```python
from build123d import *

# Parameters (mm, degrees)
BOSS_EXTRUDE1_DEPTH = 48
SKETCH2_R           = 1.5
CUT_EXTRUDE1_DEPTH  = 13
SKETCH3_R           = 1.5
SKETCH3_R_2         = 3
CUT_EXTRUDE3_DEPTH  = 21
FILLET1_R           = 5
FILLET2_R           = 15


with BuildPart() as part:
    # Sketch1 → Boss-Extrude1 (new body)
    with BuildSketch(Plane(origin=(0, 0, 0), x_dir=(1, 0, 0), z_dir=(0, 1, 0))):
        Polygon((0, 0), (0, 12), (1.5, 12), (1.5, 1.5), (20, 1.5), (20, 0), align=None)
    extrude(amount=BOSS_EXTRUDE1_DEPTH)

    # Sketch2 → Cut-Extrude1 (cut, through all)
    with BuildSketch(Plane.XY):
        with Locations((13, 31.5)):
            Circle(SKETCH2_R)
        with Locations((13, 16.5)):
            Circle(SKETCH2_R)
    extrude(amount=-CUT_EXTRUDE1_DEPTH, mode=Mode.SUBTRACT)

    # Sketch3 → Cut-Extrude3 (cut, through all)
    with BuildSketch(Plane(origin=(0, 0, 0), x_dir=(0, 0, -1), z_dir=(1, 0, 0))):
        with Locations((7, 42)):
            Circle(SKETCH3_R)
        with Locations((7, 24)):
            Circle(SKETCH3_R_2)
        with Locations((7, 6)):
            Circle(SKETCH3_R)
    extrude(amount=CUT_EXTRUDE3_DEPTH, mode=Mode.SUBTRACT)

    # Fillet1
    fillet1_edges = [part.edges().sort_by_distance(p)[0] for p in [
        (0.75, 48, -12),
        (0.75, 0, -12),
    ]]
    fillet(fillet1_edges, radius=FILLET1_R)

    # Fillet2
    fillet2_edges = [part.edges().sort_by_distance(p)[0] for p in [
        (20, 48, -0.75),
        (20, 0, -0.75),
    ]]
    fillet(fillet2_edges, radius=FILLET2_R)


solid = part.part
```
Verification items for the finished model (mm, model axes). A direction names the side the tool comes from. Coordinates: 2 decimals unless noted, no trailing zeros. Write each loop counter-clockwise with the first axis right and the second up, starting at its lowest first coordinate (ties: lowest second). Pieces come first, ordered by that corner, then holes. Notation, with made-up numbers: M 6,-4.75 L 45,-4.75 A28 cw 45,22.25 Z; hole C 75.25,-7 d1. An arc over 180 degrees is marked long. One line per item, written item: value.
Item 1: Section check A-A, the plane y = 31.5. Record the boundary of the cut face in (x, z), plus the area to 4 significant figures.
Check sheet entries:
outline: M 0,-12 L 1.5,-12 L 1.5,-1.5 L 11.5,-1.5 L 11.5,0 L 0,0 Z; M 14.5,-1.5 L 20,-1.5 L 20,0 L 14.5,0 Z
area: 41.25 mm^2
Item 2: Mould release check, pull along Z, two halves, no side actions. Record for faces 1 (the flat face through (11, 24, -1.5)), 2 (the cylindrical face through (0.74, 40.536, -6.675)), 3 (the cylindrical face through (15.49, 43.72, -0.74)): pulls with the +Z half, pulls with the -Z half, needs draft (parallel to the pull), parting line crosses it, or undercut.
Check sheet entries:
face 1: pulls with the -Z half
face 2: undercut
face 3: needs draft
Item 3: Gauge pin test, flat ends, axial feed: pin 1 Ø12 at (x, y) = (11, 26) entering from -Z; pin 2 Ø1.5 at (x, z) = (3.5, -9) entering from +Y; pin 3 Ø5 at (y, z) = (35, -6) entering from +X. Record the tip position at first contact, or that the pin passes through.
Check sheet entries:
pin 1: stops at z = -1.5
pin 2: passes through
pin 3: stops at x = 1.5
Item 4: Section check B-B, the plane x = 13. Record the boundary of the cut face in (y, z), plus the area to 3 significant figures.
Check sheet entries:
outline: M 2.31,-1.5 L 15,-1.5 L 15,0 L 2.31,0 Z; M 18,-1.5 L 30,-1.5 L 30,0 L 18,0 Z; M 33,-1.5 L 45.69,-1.5 L 45.69,0 L 33,0 Z
area: 56.1 mm^2
Item 5: Access from +Z, -Z, +X, -X, +Y, -Y to the whole of each face (thin tool, end or side, straight path). Record for faces 4 (the cylindrical face through (1, 1, -10)), 5 (the flat face through (1.5, 24, -3)).
Check sheet entries:
face 4: -Z, +X, -X, -Y
face 5: -Z, +X, +Y, -Y
Item 6: Scan lines: line 1 along Y through (x, z) = (0.7, -7); line 2 along Y through (x, z) = (1, -8.25); line 3 along Y through (x, z) = (13, -0.55). Record each from-to range of solid material in increasing order.
Check sheet entries:
line 1: y = 0 to 4.5, 7.5 to 21, 27 to 40.5, 43.5 to 48
line 2: y = 0.16 to 5.17, 6.83 to 21.27, 26.73 to 41.17, 42.83 to 47.84
line 3: y = 2.31 to 15, 18 to 30, 33 to 45.69
Item 7: Section check C-C, the plane z = -6. Record the boundary of the cut face in (x, y), plus the area to 3 significant figures.
Check sheet entries:
outline: M 0,0 L 1.5,0 L 1.5,4.88 L 0,4.88 Z; M 0,7.12 L 1.5,7.12 L 1.5,21.17 L 0,21.17 Z; M 0,26.83 L 1.5,26.83 L 1.5,40.88 L 0,40.88 Z; M 0,43.12 L 1.5,43.12 L 1.5,48 L 0,48 Z
area: 56.8 mm^2
Item 8: Section check D-D, the plane y = 6. Record the boundary of the cut face in (x, z).
Check sheet entries:
outline: M 0,-12 L 1.5,-12 L 1.5,-8.5 L 0,-8.5 Z; M 0,-5.5 L 1.5,-5.5 L 1.5,-1.5 L 17,-1.5 L 17,0 L 0,0 Z
